Here's how the part is built. I have some questions about the finished solid (model axes, mm). A direction names the side the tool comes from. Coordinates: 2 decimals unless noted, no trailing zeros. Loops run counter-clockwise (first coordinate to the right, second up) from the corner with the lowest first, then second, coordinate; pieces in that order, holes last. Notation, with made-up numbers: (-0.5, 44) -> (30.5, 44) arc R17 cw to (30.5, 57) -> close; hole circle Ø2 at (68, -36). An arc over 180 degrees is marked (long way). Use CSV: the item, a comma, the result in double quotes. Start each with the question number.
from build123d import *

# Parameters (mm, degrees)
BOSS_EXTRUDE2_DEPTH = 1.58
CUT_EXTRUDE4_DEPTH  = 49.333297529
SKETCH6_R           = 0.3
CUT_EXTRUDE9_DEPTH  = 49.333297529
SKETCH5_R           = 0.3
SKETCH5_R_2         = 1.525
CUT_EXTRUDE10_DEPTH = 49.333297529
SKETCH7_R           = 0.65
SKETCH7_R_2         = 0.495
SKETCH7_R_3         = 0.3
SKETCH7_R_4         = 1.625
SKETCH7_R_5         = 1.375
CUT_EXTRUDE11_DEPTH = 49.333297529
SKETCH13_R          = 2
CUT_EXTRUDE12_DEPTH = 49.333297529


with BuildPart() as part:
    # Sketch3 → Boss-Extrude2 (new body)
    with BuildSketch(Plane.XY):
        with BuildLine():
            Line((-38.533712153, -25.825), (38.533712153, -25.825))
            ThreePointArc((38.533712153, -25.825), (39.08143471, -25.661660027), (39.450227292, -25.225))
            ThreePointArc((39.450227292, -25.225), (39.764339828, -24.764339828), (40.225, -24.450227292))
            ThreePointArc((40.225, -24.450227292), (40.661660027, -24.08143471), (40.825, -23.533712153))
            Line((40.825, -23.533712153), (40.825, 23.533712153))
            ThreePointArc((40.825, 23.533712153), (40.661660027, 24.08143471), (40.225, 24.450227292))
            ThreePointArc((40.225, 24.450227292), (39.764339828, 24.764339828), (39.450227292, 25.225))
            ThreePointArc((39.450227292, 25.225), (39.08143471, 25.661660027), (38.533712153, 25.825))
            Line((38.533712153, 25.825), (-38.533712153, 25.825))
            ThreePointArc((-38.533712153, 25.825), (-39.08143471, 25.661660027), (-39.450227292, 25.225))
            ThreePointArc((-39.450227292, 25.225), (-39.764339828, 24.764339828), (-40.225, 24.450227292))
            ThreePointArc((-40.225, 24.450227292), (-40.661660027, 24.08143471), (-40.825, 23.533712153))
            Line((-40.825, 23.533712153), (-40.825, -23.533712153))
            ThreePointArc((-40.825, -23.533712153), (-40.661660027, -24.08143471), (-40.225, -24.450227292))
            ThreePointArc((-40.225, -24.450227292), (-39.764339828, -24.764339828), (-39.450227292, -25.225))
            ThreePointArc((-39.450227292, -25.225), (-39.08143471, -25.661660027), (-38.533712153, -25.825))
        make_face()
    extrude(amount=BOSS_EXTRUDE2_DEPTH)

    # Sketch8 → Cut-Extrude4 (cut, through all)
    with BuildSketch(Plane.XY.offset(1.58)):
        with BuildLine():
            Line((10.592557127, 25.825), (10.592557127, 15.905077804))
            ThreePointArc((10.592557127, 15.905077804), (14.134043321, 12.36359161), (17.675529515, 15.905077804))
            Line((17.675529515, 15.905077804), (17.675529515, 25.825))
            Line((17.675529515, 25.825), (10.592557127, 25.825))
        make_face()
    extrude(amount=-CUT_EXTRUDE4_DEPTH, mode=Mode.SUBTRACT)

    # Sketch6 → Cut-Extrude9 (cut, through all)
    with BuildSketch(Plane.XY.offset(1.58)):
        with Locations((-19.175, 16.525)):
            Circle(SKETCH6_R)
        with Locations((-19.175, 4.925)):
            Circle(SKETCH6_R)
    extrude(amount=-CUT_EXTRUDE9_DEPTH, mode=Mode.SUBTRACT)

    # Sketch5 → Cut-Extrude10 (cut, through all)
    with BuildSketch(Plane(origin=(0, 0, 0), x_dir=(1, 0, 0), z_dir=(0, 0, -1))):
        with Locations((-19.175, -4.925)):
            Circle(SKETCH5_R)
        with Locations((-19.175, -16.525)):
            Circle(SKETCH5_R)
        with Locations(Location((-21.945, -22.525, 0), (0, 0, 180))):
            Circle(SKETCH5_R_2)
        with Locations(Location((-21.945, 1.075, 0), (0, 0, 180))):
            Circle(SKETCH5_R_2)
    extrude(amount=-CUT_EXTRUDE10_DEPTH, mode=Mode.SUBTRACT)

    # Sketch7 → Cut-Extrude11 (cut, through all)
    with BuildSketch(Plane(origin=(0, 0, 0), x_dir=(1, 0, 0), z_dir=(0, 0, -1))):
        with Locations(Location((-36.578389688, 20.415177754, 0), (0, 0, 270))):
            Circle(SKETCH7_R)
        with Locations(Location((-29.568389688, 20.415177754, 0), (0, 0, 270))):
            Circle(SKETCH7_R)
        with Locations(Location((-35.323389688, 22.905177754, 0), (0, 0, 270))):
            Circle(SKETCH7_R_2)
        with Locations(Location((-30.823389688, 22.905177754, 0), (0, 0, 270))):
            Circle(SKETCH7_R_2)
        with Locations(Location((-35.839874228, -12.060017363, 0), (0, 0, 270))):
            Circle(SKETCH7_R_3)
        with Locations(Location((-31.810125772, -16.157982637, 0), (0, 0, 270))):
            Circle(SKETCH7_R_3)
        with Locations(Location((31.286432501, -16.58, 0), (0, 0, 270))):
            Circle(SKETCH7_R_4)
        with Locations(Location((37.283538512, -16.58, 0), (0, 0, 270))):
            Circle(SKETCH7_R_5)
        with Locations(Location((34.3, -11.85761971, 0), (0, 0, 270))):
            Circle(SKETCH7_R_5)
        with Locations(Location((37.12, -7.675, 0), (0, 0, 270))):
            Circle(SKETCH7_R_4)
        with Locations(Location((37.12, 3.755, 0), (0, 0, 270))):
            Circle(SKETCH7_R_4)
        with Locations(Location((37.12, 8.065, 0), (0, 0, 270))):
            Circle(SKETCH7_R_4)
        with Locations(Location((37.12, 19.495, 0), (0, 0, 270))):
            Circle(SKETCH7_R_4)
    extrude(amount=-CUT_EXTRUDE11_DEPTH, mode=Mode.SUBTRACT)

    # Sketch13 → Cut-Extrude12 (cut, through all)
    with BuildSketch(Plane.XY.offset(1.58)):
        with Locations((-28.825, 25.825)):
            Circle(SKETCH13_R)
    extrude(amount=-CUT_EXTRUDE12_DEPTH, mode=Mode.SUBTRACT)


solid = part.part
1) I want a section at B-B, the plane z = 1.2. State how many separate pieces and enclosed holes the cut face has, plus the area to 3 significant figures.
2) Please list where these lines run through material, in increasing order: L1, parallel to X at y = -23, z = 0.75 (3 decimals); L2, parallel to X at y = 16, z = 1.15 (3 decimals); L3, parallel to Y at x = 32, z = 1.35 (3 decimals). Write a range as [from, to].
3) For P1, Ø1, axis at x = -36.58, y = -20.42, coming from the +Z side, with a flat end and sliding along its axis, tell me the tip position at first contact or that it passes through.
4) I want a section at A-A, the plane x = 34.3. Please give me the cut outline in (y, z) (3 decimals), plus the area to 3 significant figures.
5) Which directions (+Z, -Z, +X, -X, +Y, -Y) give clear straight access to the entire face, cutting with the end or side of a thin tool? Please do faces 5 (the face through (-35, 25.825, 1)), 6 (the face through (10.593, 21, 1)).
6) Thinking about a two-plate mould opening in Y: for faces 1 (the face through (-28.869, 23.825, 0.801)), 2 (the face through (-1, 0, 1.58)), 3 (the face through (-1, -25.825, 1)), 4 (the face through (35.534, -4.107, 0.779)), which applies, pulls with the +Y half, pulls with the -Y half, needs draft (parallel to the pull), parting line crosses it, or undercut?
Return value:
1,separate pieces,"1"
1,enclosed holes,"17"
1,area,"4,040 mm²"
2,L1,"x = [-40.825, -35.809], [-34.838, -31.309], [-30.338, 40.825]"
2,L2,"x = [-40.825, -32.065], [-31.555, 10.593], [17.676, 29.768], [32.804, 36.037], [38.53, 40.825]"
2,L3,"y = [-25.825, 15.12], [18.04, 25.825]"
3,P1,"passes through"
4,outline,"(-25.825, 0) -> (10.483, 0) -> (10.483, 1.58) -> (-25.825, 1.58) -> close; (13.233, 0) -> (25.825, 0) -> (25.825, 1.58) -> (13.233, 1.58) -> close"
4,area,"77.3 mm²"
5,face 5,"+Z, -Z, +X, -X, +Y"
5,face 6,"+Z, -Z, +Y"
6,face 1,"pulls with the +Y half"
6,face 2,"needs draft"
6,face 3,"pulls with the -Y half"
6,face 4,"undercut"
